```python
from build123d import *

# Parameters (mm, degrees)
F0_R     = 0.15
F1_DEPTH = 2.5
F2_R     = 1.5
F3_DEPTH = 2.4
F5_DEPTH = 25
F7_DEPTH = 25
F8_R     = 2
F9_SIZE  = 0.25


with BuildPart() as f1:
    # F0 (on Right) → F1 (new body)
    with BuildSketch(Plane.YZ):
        with BuildLine():
            ThreePointArc((-3.1, 0), (-1.55, -1.55), (0, 0))
            Line((0, 0), (0, 20))
            ThreePointArc((0, 20), (-1.55, 21.55), (-3.1, 20))
            Line((-3.1, 20), (-3.1, 0))
        make_face()
        with Locations((-1.55, 17.244)):
            Circle(F0_R, mode=Mode.SUBTRACT)
        with Locations((-1.55, 18.644)):
            Circle(F0_R, mode=Mode.SUBTRACT)
    extrude(amount=F1_DEPTH)

    # F2 (on face) → F3 (join)
    with BuildSketch(Plane.YZ.offset(2.5)):
        with Locations((-1.55, 0)):
            Circle(F2_R)
    extrude(amount=F3_DEPTH)

    # F4 (on face) → F5 (cut)
    with BuildSketch(Plane.XZ.offset(3.1)):
        Polygon((2.5, 10.55), (2.5, 21.55), (1, 21.55), (1, 10.55), (2.5, 2.0031642634), align=None)
    extrude(amount=-F5_DEPTH, mode=Mode.SUBTRACT)

    # F6 (on face) → F7 (cut)
    with BuildSketch(Plane.XZ.offset(3.1)):
        Polygon((1.6280860873, 2.0031642634), (0, 10.55), (0, -2.1245246753), (1.6280860873, -2.1245246753), align=None)
    extrude(amount=-F7_DEPTH, mode=Mode.SUBTRACT)

    # F8
    f8_edges = [f1.edges().sort_by_distance(p)[0] for p in [
        (1, -1.55, 10.55),
        (2.5, -1.55, 2.003164),
        (1.628086, -1.55, 2.003164),
        (0, -1.55, 10.55),
    ]]
    fillet(f8_edges, radius=F8_R)

    # F9
    f9_edges = [f1.edges().sort_by_distance(p)[0] for p in [
        (4.9, -3.05, 0),
    ]]
    chamfer(f9_edges, length=F9_SIZE)


solid = f1.part
```
Read the model definition and answer for the solid it produces. Units are mm, in the model's axes. A direction names the side the tool comes from. Round coordinates to 2 decimals unless told otherwise and drop trailing zeros. Write each loop counter-clockwise with the first axis right and the second up, starting at its lowest first coordinate (ties: lowest second). Pieces come first, ordered by that corner, then holes. Notation, with made-up numbers: (-30.5, 38.25) -> (21.5, 38.25) arc R18 cw to (21.5, 43.25) -> close; hole circle Ø9 at (49.5, -27.75). An arc over 180 degrees is marked (long way). Answer in a Markdown table with one row per item. Add a question column.
1) Find section A-A, the plane x = 0.45. Determine the outline of the cut face in (y, z).
2) Consider line 1 (X direction, y = -2.6, z = 17.25); line 2 (X direction, y = -2.2, z = 1); line 3 (Z direction, x = 4.5, y = -1.55). Determine where each line is inside the solid, lowest interval first.
3) Which of the six approach directions +Z, -Z, +X, -X, +Y, -Y give full straight-line access (tool end or side, diameter ignored) to faces 1 (the face through (2.5, -1.44, 1.65)), 2 (the face through (1, -2, 16)), 3 (the face through (1.628, -2, 0)), 4 (the face through (0.95, 0, 9.86)), 5 (the face through (2.06, -1.58, -1.55))?
4) Find section C-C, the plane x = 3.85. Determine the outline of the cut face in (y, z), and give its area (3 significant figures).
5) Find section B-B, the plane z = 13. Determine the outline of the cut face in (x, y), and give its area (3 significant figures).
6) Find section D-D, the plane z = 3.5. Determine the outline of the cut face in (x, y).
7) Given P1, Ø1.5, axis at y = -2, z = 16.5, coming from the +X side, flat-ended and moving along its own axis, determine where the tip first touches the part or whether it passes through.
Findings below:
| question | item | result |
|---|---|---|
| 1 | outline | (-3.1, 8.19) -> (0, 8.19) -> (0, 20) arc R1.55 ccw to (-3.1, 20) -> close; hole circle Ø0.3 at (-1.55, 17.24); hole circle Ø0.3 at (-1.55, 18.64) |
| 2 | line 1 | 0 to 1 |
| 2 | line 2 | 1.63 to 4.9 |
| 2 | line 3 | -1.5 to 1.5 |
| 3 | face 1 | +X |
| 3 | face 2 | +Z, +X, +Y, -Y |
| 3 | face 3 | -Z, -X, +Y, -Y |
| 3 | face 4 | +Z, -Z, +X, -X, +Y |
| 3 | face 5 | -Z, +X, -X |
| 4 | outline | circle Ø3 at (-1.55, 0) |
| 4 | area | 7.07 mm² |
| 5 | outline | (0, -3.1) -> (1, -3.1) -> (1, 0) -> (0, 0) -> close |
| 5 | area | 3.10 mm² |
| 6 | outline | (1.34, -3.1) -> (2.24, -3.1) -> (2.24, 0) -> (1.34, 0) -> close |
| 7 | P1 | x = 1 |
